Answer from the drawing. Dimensions are ordinates in mm from the lowest x, y and z of the part. Round coordinates to 2 decimals unless told otherwise and drop trailing zeros. Write each loop counter-clockwise with the first axis right and the second up, starting at its lowest first coordinate (ties: lowest second). Pieces come first, ordered by that corner, then holes. Notation, with made-up numbers: (24, 47.5) - (49, 47.5) arc R15 cw to (49, 57.5) - close; hole circle Ø4 at (42, 67.25). An arc over 180 degrees is marked (long way). Answer in a Markdown table with one row per item.
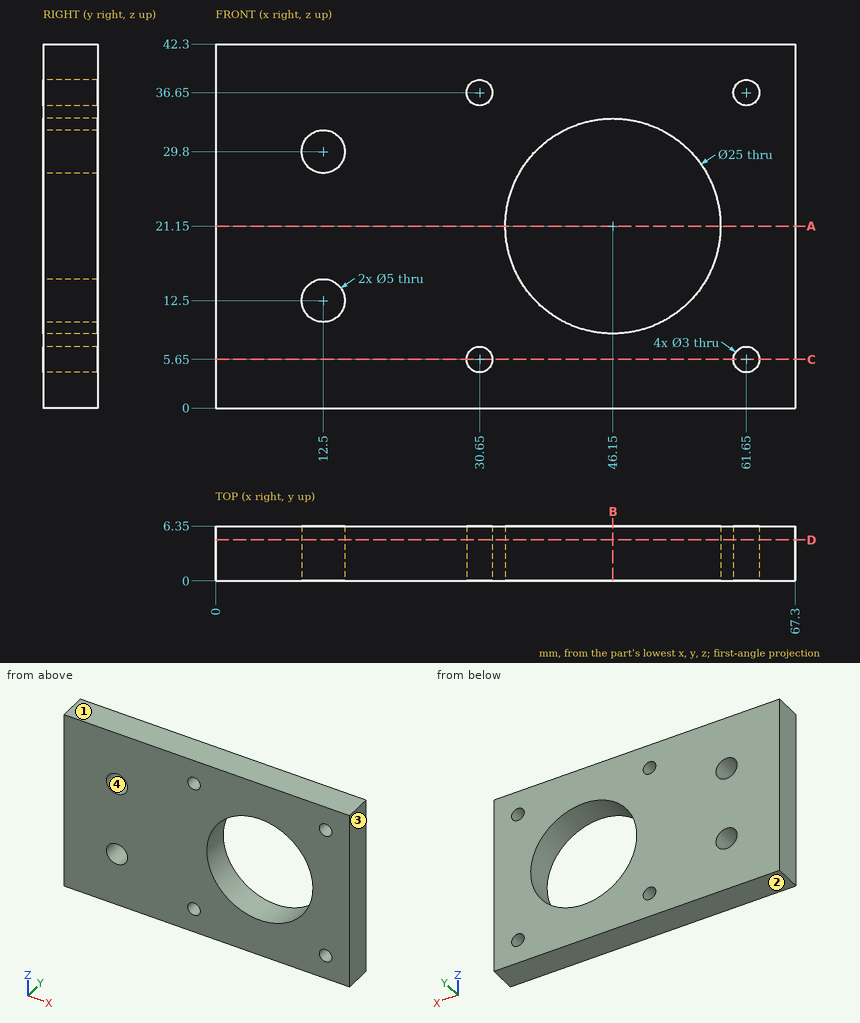
(1) For a pull along Z with two mould halves and no side action, classify the marked faces 1, 2, 3 and 4 as pulls with the +Z half, pulls with the -Z half, needs draft (parallel to the pull), parting line crosses it, or undercut.
Checked values:
| item | result |
|---|---|
| face 1 | pulls with the +Z half |
| face 2 | pulls with the -Z half |
| face 3 | needs draft |
| face 4 | undercut |
(2) Section D-D (y = 4.75) is taken. Give the vertices of the cut face in (x, z), and give its area (3 significant figures).
Checked values:
| item | result |
|---|---|
| outline | (0, 0) - (67.3, 0) - (67.3, 42.3) - (0, 42.3) - close; hole circle Ø5 at (12.5, 12.5); hole circle Ø5 at (12.5, 29.8); hole circle Ø3 at (30.65, 5.65); hole circle Ø3 at (30.65, 36.65); hole circle Ø25 at (46.15, 21.15); hole circle Ø3 at (61.65, 5.65); hole circle Ø3 at (61.65, 36.65) |
| area | 2,290 mm2 |
(3) Section B-B (x = 46.15) is taken. Give the vertices of the cut face in (y, z).
Checked values:
| item | result |
|---|---|
| outline | (0, 0) - (6.35, 0) - (6.35, 8.65) - (0, 8.65) - close; (0, 33.65) - (6.35, 33.65) - (6.35, 42.3) - (0, 42.3) - close |
(4) Section A-A (z = 21.15) is taken. Give the vertices of the cut face in (x, y).
Checked values:
| item | result |
|---|---|
| outline | (0, 0) - (33.65, 0) - (33.65, 6.35) - (0, 6.35) - close; (58.65, 0) - (67.3, 0) - (67.3, 6.35) - (58.65, 6.35) - close |
(5) A flat-ended cylindrical pin translates along its axis: pin 1 (1 mm diameter, centred on x = 56.5, z = 17.5, fed in from -Y). Find the tip coordinate at first contact, or state that the pin passes through.
Checked values:
| item | result |
|---|---|
| pin 1 | passes through |
(6) Section C-C (z = 5.65) is taken. Give the vertices of the cut face in (x, y), and give its area (3 significant figures).
Checked values:
| item | result |
|---|---|
| outline | (0, 0) - (29.15, 0) - (29.15, 6.35) - (0, 6.35) - close; (32.15, 0) - (60.15, 0) - (60.15, 6.35) - (32.15, 6.35) - close; (63.15, 0) - (67.3, 0) - (67.3, 6.35) - (63.15, 6.35) - close |
| area | 389 mm2 |
(7) Find the intervals of material crossed by line 1 (X direction, y = 2, z = 36.65); line 2 (Z direction, x = 31, y = 1); line 3 (X direction, y = 2.25, z = 30.5), in increasing order.
Checked values:
| item | result |
|---|---|
| line 1 | x = 0 to 29.15, 32.15 to 60.15, 63.15 to 67.3 |
| line 2 | z = 0 to 4.19, 7.11 to 35.19, 38.11 to 42.3 |
| line 3 | x = 0 to 10.1, 14.9 to 37.85, 54.45 to 67.3 |
